```python
from build123d import *

# Parameters (mm, degrees)
F1_DEPTH  = 2
F3_DEPTH  = 166
F5_D      = 5
F5_DEPTH  = 10
F7_DEPTH  = 2
F8_R      = 2
F10_DEPTH = 25
F12_DEPTH = 10
F14_DEPTH = 1
F16_DEPTH = 1


with BuildPart() as f1:
    # F0 (on Top) → F1 (new body)
    with BuildSketch(Plane.XY):
        Polygon((-42.839942, -39.786562), (18.198534, -39.786562), (10.160058, -9.786562), (-12.839942, -9.786562), (-12.839942, 20.213438), (-42.839942, 20.213438), (-42.839942, -9.786562), align=None)
    extrude(amount=F1_DEPTH)

    # F2 (on face) → F3 (join)
    with BuildSketch(Plane.XY.offset(2)):
        Polygon((-36.539942, 16.213438), (-36.539942, 18.213438), (-14.839942, 18.213438), (-14.839942, -11.786562), (8.625404, -11.786562), (15.592083, -37.786562), (-36.539942, -37.786562), (-36.539942, -35.786562), (-38.539942, -35.786562), (-38.539942, -37.786562), (-40.839942, -37.786562), (-40.839942, -35.786562), (-42.839942, -35.786562), (-42.839942, -39.786562), (18.198534, -39.786562), (10.160058, -9.786562), (-12.839942, -9.786562), (-12.839942, 20.213438), (-42.839942, 20.213438), (-42.839942, 16.213438), (-40.839942, 16.213438), (-40.839942, 18.213438), (-38.539942, 18.213438), (-38.539942, 16.213438), align=None)
    extrude(amount=F3_DEPTH)

    # F5
    with Locations(Plane(origin=(7.032822, 1.884439, 0), x_dir=(-0.258819, 0.965926, 0), z_dir=(0.965926, 0.258819, 0))):
        with Locations((-27.611852, 155), (-27.611852, 127), (-27.611852, 99), (-27.611852, 71), (-27.611852, 43), (-27.611852, 15)):
            Hole(F5_D / 2, depth=F5_DEPTH)

    # F6 (on face) → F7 (join)
    with BuildSketch(Plane.XY.offset(168)):
        Polygon((-38.539942, -39.786562), (18.198534, -39.786562), (10.160058, -9.786562), (-12.839942, -9.786562), (-12.839942, 20.213438), (-38.539942, 20.213438), (-38.539942, -37.786562), align=None)
    extrude(amount=F7_DEPTH)

    # F8
    f8_edges = [f1.edges().sort_by_distance(p)[0] for p in [
        (-12.320704, -39.786562, 0),
        (18.198534, -39.786562, 85),
        (14.179296, -24.786562, 0),
        (-10.170704, -39.786562, 170),
        (14.179296, -24.786562, 170),
    ]]
    fillet(f8_edges, radius=F8_R)

    # F9 (on face) → F10 (cut)
    with BuildSketch(Plane(origin=(0, 0, 0), x_dir=(1, 0, 0), z_dir=(0, 0, -1))):
        with BuildLine():
            ThreePointArc((-39.839942, -8.775018), (-38.425729, -8.189231), (-37.839942, -6.775018))
            ThreePointArc((-37.839942, -6.775018), (-38.425729, -5.360804), (-39.839942, -4.775018))
            ThreePointArc((-39.839942, -4.775018), (-41.839942, -6.775018), (-39.839942, -8.775018))
        make_face()
        with BuildLine():
            ThreePointArc((-39.839942, -8.775018), (-41.839942, -6.775018), (-39.839942, -4.775018))
            Line((-39.839942, -4.775018), (-42.839942, -4.775018))
            Line((-42.839942, -4.775018), (-42.839942, -8.775018))
            Line((-42.839942, -8.775018), (-39.839942, -8.775018))
        make_face()
    extrude(amount=-F10_DEPTH, mode=Mode.SUBTRACT)

    # F11 (on face) → F12 (join)
    with BuildSketch(Plane(origin=(-14.839942, 0, 0), x_dir=(0, -1, 0), z_dir=(-1, 0, 0))):
        Polygon((3.486562, 44.687904), (1.486562, 44.687904), (1.486562, 42.687904), (-0.513438, 42.687904), (-0.513438, 40.687904), (3.486562, 40.687904), align=None)
        Polygon((-16.213438, 42.687904), (-16.213438, 44.687904), (-18.213438, 44.687904), (-18.213438, 40.687904), (-14.213438, 40.687904), (-14.213438, 42.687904), align=None)
        Polygon((-16.213438, 83.787904), (-16.213438, 85.787904), (-14.213438, 85.787904), (-14.213438, 87.787904), (-18.213438, 87.787904), (-18.213438, 83.787904), align=None)
        Polygon((-0.513438, 87.787904), (-0.513438, 85.787904), (1.486562, 85.787904), (1.486562, 83.787904), (3.486562, 83.787904), (3.486562, 87.787904), align=None)
    extrude(amount=F12_DEPTH)

    # F13 (on face) → F14 (cut)
    with BuildSketch(Plane.XY.offset(2)):
        Polygon((14.556807, -37.786562), (7.590128, -11.786562), (-14.839942, -11.786562), (-14.839942, -37.786562), align=None)
    extrude(amount=-F14_DEPTH, mode=Mode.SUBTRACT)

    # F15 (on face) → F16 (cut)
    with BuildSketch(Plane(origin=(0, 0, 168), x_dir=(1, 0, 0), z_dir=(0, 0, -1))):
        Polygon((-14.839942, 11.786562), (7.590128, 11.786562), (14.556807, 37.786562), (-14.839942, 37.786562), align=None)
    extrude(amount=-F16_DEPTH, mode=Mode.SUBTRACT)


solid = f1.part
```
Can you work these out from the model? Positions are in its coordinate system, mm. A direction names the side the tool comes from. Coordinates: 2 decimals unless noted, no trailing zeros. Loops run counter-clockwise (first coordinate to the right, second up) from the corner with the lowest first, then second, coordinate; pieces in that order, holes last. Notation, with made-up numbers: M -4,57.5 L 50,57.5 A24 ccw 50,76.5 Z; hole C -36.75,54 d9. An arc over 180 degrees is marked long. Put each result on its own line as item: value. Start each with the question number.
(1) Which directions (+Z, -Z, +X, -X, +Y, -Y) give clear straight access to the entire face, cutting with the end or side of a thin tool? Please do faces 5 (the face through (-24.84, -2, 42)), 6 (the face through (-12.84, 5, 84)), 7 (the face through (0, -25, 1)), 8 (the face through (-38.54, 17, 86)).
(2) Will these pins go through, and if not, where does the flat tip stop? pin 1 Ø18 at (y, z) = (-20, 81) entering from -X; pin 2 Ø3 at (y, z) = (4, 80.5) entering from +X; pin 3 Ø0.6 at (y, z) = (-37, 98.5) entering from +X.
(3) We'd pull the mould along X, two halves only. Please class faces 1 (the face through (-26, 18.213, 84)), 2 (the face through (-42.84, 18, 84)), 3 (the face through (-28, 20.213, 84)), 4 (the face through (13.5, -26.2, 68.8)): +X half, -X half, draft (parallel to the pull), parting line (faces both ways), or undercut.
(4) I need wall thicknesses on probe 1 along X at (y, z) = (17, 124.5); probe 2 along Y at (x, z) = (-3.5, 123); probe 3 along Z at (x, y) = (-15.5, 12.5). Which ranges of each line are inside material? Lowest first, please.
(5) Imagine slicing it at B-B on x = -29. List the corners of the cut face in (y, z) for me, and give its area (3 significant figures).
(6) Imagine slicing it at A-A on x = -16.5. Give the number of separate pieces and of enclosed holes in the cut face, and give its area (3 significant figures).
(7) Imagine slicing it at D-D on x = 1. List the corners of the cut face in (y, z) for me.
(8) Imagine slicing it at C-C on z = 23. List the corners of the cut face in (x, y) for me.
Worked answers:
1. face 5: -X
1. face 6: +Z, -Z, +X, +Y
1. face 7: none
1. face 8: +Z
2. pin 1: stops at x = -14.84
2. pin 2: stops at x = -12.84
2. pin 3: stops at x = 17.53
3. face 1: undercut
3. face 2: -X half
3. face 3: draft
3. face 4: parting line
4. probe 1: x = -42.84 to -40.84, -38.54 to -36.54, -14.84 to -12.84
4. probe 2: y = -39.79 to -37.79, -11.79 to -9.79
4. probe 3: z = 0 to 2, 168 to 170
5. outline: M -39.79,2 A2 ccw -37.79,0 L 20.21,0 L 20.21,170 L -37.79,170 A2 ccw -39.79,168 Z; hole M -37.79,2 L 18.21,2 L 18.21,168 L -37.79,168 Z
5. area: 902 mm2
6. separate pieces: 3
6. enclosed holes: 1
6. area: 950 mm2
7. outline: M -39.79,2 A2 ccw -37.79,0 L -9.79,0 L -9.79,170 L -37.79,170 A2 ccw -39.79,168 Z; hole M -37.79,1 L -11.79,1 L -11.79,169 L -37.79,169 Z
8. outline: M -42.84,-39.79 L 15.59,-39.79 A2 ccw 17.52,-37.27 L 10.16,-9.79 L -12.84,-9.79 L -12.84,20.21 L -42.84,20.21 L -42.84,16.21 L -40.84,16.21 L -40.84,18.21 L -38.54,18.21 L -38.54,16.21 L -36.54,16.21 L -36.54,18.21 L -14.84,18.21 L -14.84,-11.79 L 8.63,-11.79 L 15.59,-37.79 L -36.54,-37.79 L -36.54,-35.79 L -38.54,-35.79 L -38.54,-37.79 L -40.84,-37.79 L -40.84,-35.79 L -42.84,-35.79 Z
